Source: CAD feature listing. Evaluate the final solid. Frame: model axes, mm. Face numbers are marked on the shaded views. A direction names the side the tool comes from. Round coordinates to 2 decimals unless told otherwise and drop trailing zeros. Write each loop counter-clockwise with the first axis right and the second up, starting at its lowest first coordinate (ties: lowest second). Pieces come first, ordered by that corner, then holes.
Autodesk Inventor part; units mm, degrees
ref_plane "body_screw_XY" through (0, -9, 3) normal (0, 0, 1) x (1, 0, 0)
ref_plane "body_screw_YZ" through (0, -9, 3) normal (1, 0, 0) x (0, 1, 0)
ref_plane "body_screw_ZX" through (0, -9, 3) normal (0, 1, 0) x (0, 0, 1)
sketch "Sketch_1" plane through (0, 0, 0) normal (0, 0, 1) x (1, 0, 0)
  line L0 (3, 0) -> (-3, 0)
  line L1 (-3, 12) -> (-3, 6.5)
  line L2 (-3, 6.5) -> (-2.5, 6)
  line L3 (-2.5, 6) -> (2.5, 6)
  line L4 (2.5, 6) -> (3, 6.5)
  line L5 (3, 6.5) -> (3, 12)
  line L6 (3, 12) -> (2.5, 12.5)
  line L7 (2.5, 12.5) -> (-2.5, 12.5)
  line L8 (-2.5, 12.5) -> (-3, 12)
revolve "Revolution1" add sketch "Sketch_1" angle 360 about axis through (3, 0, 0) along (1, 0, 0)
sketch "Sketch_2" plane through (0, 0, 0) normal (1, 0, 0) x (0, 1, 0)
  line L0 (-12.5, 0.75) -> (-12.5, -0.75)
  line L1 (-12.5, -0.75) -> (9, -0.75)
  line L2 (9, -0.75) -> (9, 0.75)
  line L3 (9, 0.75) -> (-12.5, 0.75)
extrude "Extrusion1" cut sketch "Sketch_2" along normal mid plane 6
sketch "Sketch_3" plane through (0, 0, 0) normal (1, 0, 0) x (0, 1, 0)
  line L0 (-9, 12.5) -> (-9, 0)
  line L1 (-9, 0) -> (-10.45, 0)
  line L2 (-10.45, 0) -> (-10.45, 3)
  line L3 (-10.45, 3) -> (-11.45, 3)
  line L4 (-11.45, 3) -> (-11.45, 12.5)
  line L5 (-11.45, 12.5) -> (-9, 12.5)
  line L6 (-9, 12.5) -> (-9, 0)
revolve "Revolution2" cut sketch "Sketch_3" angle 360 about axis through (0, -9, 12.5) along (0, 0, 1)
sketch "Sketch_4" plane through (0, 0, 0) normal (1, 0, 0) x (0, 1, 0)
  line L0 (-9, -14.25) -> (-9, -0.75)
  line L1 (-9, -0.75) -> (-7.75, -0.75)
  line L2 (-7.75, -0.75) -> (-7.9935, -0.9935)
  line L3 (-7.9935, -0.9935) -> (-7.9935, -14.25)
  line L4 (-7.9935, -14.25) -> (-9, -14.25)
  line L5 (-9, -14.25) -> (-9, -0.75)
revolve "Revolution3" cut sketch "Sketch_4" angle 360 about axis through (0, -9, -14.25) along (0, 0, -1)
thread "Thread1"
sketch "Sketch_7" plane through (0, 0, -9.5) normal (0, 0, 1) x (1, 0, 0)
  line L0 (3, 0) -> (-3, 0)
  line L1 (-3, 0) -> (-3, 1.5)
  line L2 (-3, 1.5) -> (-2.7295, 1.2295)
  line L3 (-2.7295, 1.2295) -> (2.7295, 1.2295)
  line L4 (2.7295, 1.2295) -> (3, 1.5)
  line L5 (3, 1.5) -> (3, 0)
  line L6 (3, 0) -> (-3, 0)
revolve "Revolution4" cut sketch "Sketch_7" angle 360 about axis through (3, 0, -9.5) along (1, 0, 0)
thread "Thread2"
sketch "Sketch_8" plane through (0, 0, 9.5) normal (0, 0, 1) x (1, 0, 0)
  line L0 (3, 0) -> (-3, 0)
  line L1 (-3, 0) -> (-3, 1.5)
  line L2 (-3, 1.5) -> (-2.7295, 1.2295)
  line L3 (-2.7295, 1.2295) -> (2.7295, 1.2295)
  line L4 (2.7295, 1.2295) -> (3, 1.5)
  line L5 (3, 1.5) -> (3, 0)
  line L6 (3, 0) -> (-3, 0)
revolve "Revolution5" cut sketch "Sketch_8" angle 360 about axis through (3, 0, 9.5) along (1, 0, 0)
thread "Thread3"
ref_plane "body_screw_XY" through (0, -9, 3) normal (0, 0, 1) x (1, 0, 0)
ref_plane "body_screw_YZ" through (0, -9, 3) normal (1, 0, 0) x (0, 1, 0)
ref_plane "body_screw_ZX" through (0, -9, 3) normal (0, 1, 0) x (0, 0, 1)
properties part number "SCSWJ12-6_b"
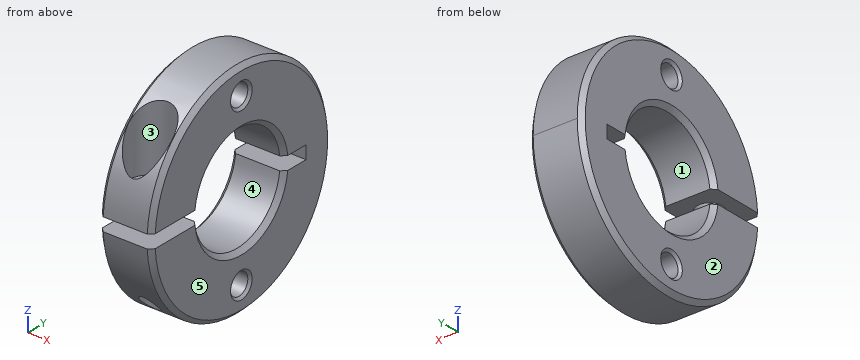
1) Material intervals for line 1 (X direction, y = -9, z = -7.5); line 2 (Y direction, x = 0.75, z = -3.5); line 3 (Y direction, x = 1.5, z = 5.5), sorted ascending.
Taken from the geometry:
line 1: x = -3 to -1.01, 1.01 to 3
line 2: y = -12 to -9.67, -8.33 to -4.87, 4.87 to 12
line 3: y = -11.22 to -10.94, -7.06 to -2.4, 2.4 to 11.22
2) Reachability of the marked faces 4 and 5 from +Z, -Z, +X, -X, +Y, -Y: full face, straight path, thin tool, end or side. Return the list, or none.
Taken from the geometry:
face 4: +X, -X
face 5: +Z, -Z, +X, +Y, -Y
3) Section query A-A on y = 0. State how many separate pieces and enclosed holes the cut face has, then the cut area to 3 significant figures.
Taken from the geometry:
separate pieces: 4
enclosed holes: 0
area: 47.2 mm2
4) Contact query for flat-ended pins moving along their axis: P1, Ø1.8, axis at x = -1, y = -8.5, coming from the +Z side; P2, Ø1.5, axis at x = 0, y = 7, coming from the -Z side; P3, Ø3, axis at x = 0, y = -9, coming from the -Z side. Output: stop coordinate, or through.
Taken from the geometry:
P1: stops at z = 3
P2: stops at z = -10.83
P3: stops at z = -10
5) Pull-direction query (Y, two-part tool) for the marked faces 1, 2 and 3; classes: released by +Y, released by -Y, zero draft, split by the parting line, or undercut.
Taken from the geometry:
face 1: undercut
face 2: zero draft
face 3: undercut
6) Section query B-B on x = 0. Return the cut outline in (y, z).
Taken from the geometry:
outline: (-12.48, -0.75) arc R12.5 ccw to (-10.01, -7.49) - (-10.01, -0.99) - (-10.25, -0.75) - close; (-12.48, 0.75) - (-10.45, 0.75) - (-10.45, 3) - (-11.45, 3) - (-11.45, 5.01) arc R12.5 ccw to start; (-7.99, -9.61) arc R12.5 ccw (long way) to (-6.55, 10.65) - (-6.55, 3) - (-7.55, 3) - (-7.55, 0.75) - (-5.95, 0.75) arc R6 cw to (5.95, 0.75) - (9, 0.75) - (9, -0.75) - (5.95, -0.75) arc R6 cw to (-5.95, -0.75) - (-7.75, -0.75) - (-7.99, -0.99) - close; hole circle Ø2.46 at (0, -9.5); hole circle Ø2.46 at (0, 9.5)
